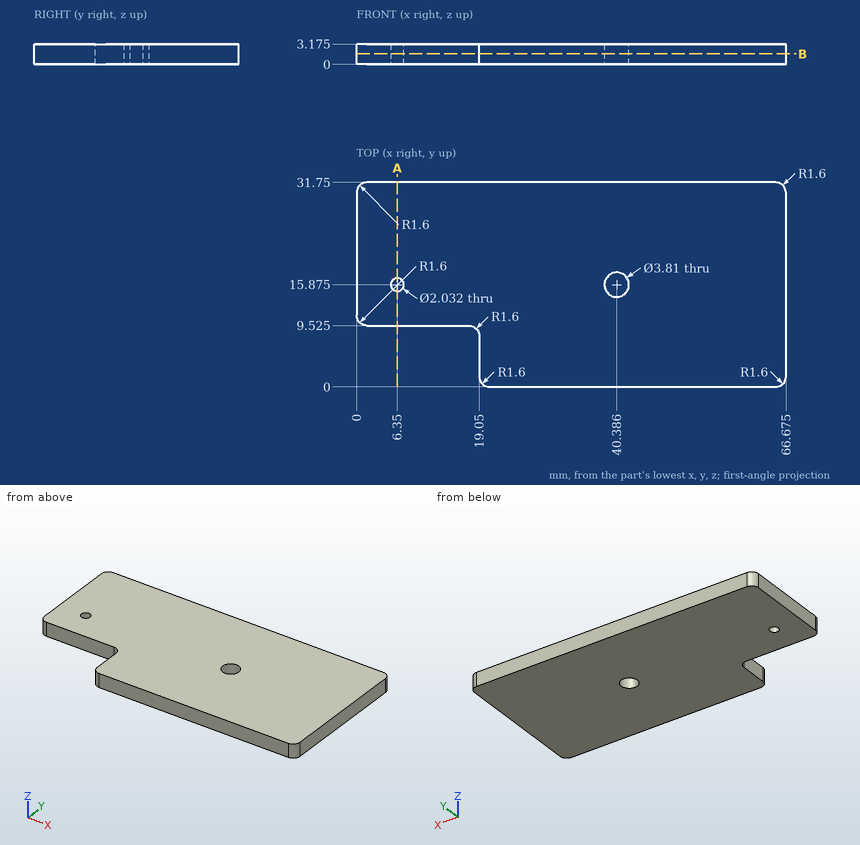
Design review of the part shown in the three views and the two pictorial views. Dimensions are in mm from the part's minimum x, y and z. Round coordinates to 2 decimals unless told otherwise and drop trailing zeros. Write each loop counter-clockwise with the first axis right and the second up, starting at its lowest first coordinate (ties: lowest second). Pieces come first, ordered by that corner, then holes. Notation, with made-up numbers: (-1.75, 8) -> (29.25, 8) arc R34 cw to (29.25, 47) -> close; hole circle Ø1 at (55, -28.75). An arc over 180 degrees is marked (long way). Answer as a JSON object with one key per item and string values.
1. Clearance check with a flat-ended pin moving along its axis: pin 1 (1 mm diameter, centred on y = 5.5, z = 2.5, fed in from -X). State where the tip first meets the part, or that it passes through.
Results found:
{"pin 1": "stops at x = 19.05"}
2. To check wall thickness, follow line 1 along Y through (x, z) = (6.35, 2) (3 decimals); line 2 along Y through (x, z) = (10.5, 2.35) (3 decimals); line 3 along X through (y, z) = (2.5, 1.6) (3 decimals). State the ranges of each line that lie inside material, in increasing order.
Results found:
{"line 1": "y = 9.525 to 14.859, 16.891 to 31.75", "line 2": "y = 9.525 to 31.75", "line 3": "x = 19.05 to 66.675"}
3. We need section A-A on x = 6.35. State the section outline as (y, z) points (3 decimals).
Results found:
{"outline": "(9.525, 0) -> (14.859, 0) -> (14.859, 3.175) -> (9.525, 3.175) -> close; (16.891, 0) -> (31.75, 0) -> (31.75, 3.175) -> (16.891, 3.175) -> close"}
4. We need section B-B on z = 1.65. State how many separate pieces and enclosed holes the cut face has, and give its area (3 significant figures).
Results found:
{"separate pieces": "1", "enclosed holes": "2", "area": "1,920 mm^2"}
